Autodesk Inventor part; units mm, degrees
ref_plane "YZ Plane" through (0, 0, 0) normal (1, 0, 0) x (0, 1, 0)
ref_plane "XZ Plane" through (0, 0, 0) normal (0, 1, 0) x (-1, 0, 0)
ref_plane "XY Plane" through (0, 0, 0) normal (0, 0, 1) x (1, 0, 0)
sketch "Skizze1" plane through (0, 0, 0) normal (0, 1, 0) x (-1, 0, 0)
  arc A0 (112.1495, -122.8972) -> (112.1495, -22.8972) centre (112.1495, -72.8972) ccw
  circle A1 centre (8.4112, -73.6215) radius 17.5
  line L0 (112.1495, -122.8972) -> (8.4112, -91.1215)
  line L1 (112.1495, -22.8972) -> (8.4112, -56.1215)
  point P0 (0, 0)
  dimension "d0" = 50
  dimension "d1" = 35
extrude "Extrusion1" add sketch "Skizze1" along normal blind 10
sketch "Skizze2" plane through (0, 10, 0) normal (0, 1, 0) x (1, 0, 0)
  arc A0 (-112.1495, 122.8972) -> (-112.1495, 22.8972) centre (-112.1495, 72.8972) ccw
  circle A1 centre (-112.1495, 72.8972) radius 40
  point P0 (0, 0)
  dimension "d4" = 80
extrude "Extrusion2" add sketch "Skizze2" along normal blind 30
sketch "Skizze3" plane through (0, 0, 0) normal (0, -1, 0) x (1, 0, 0)
  circle A0 centre (-112.1495, -112.8972) radius 2.5
  circle A1 centre (-112.1495, -32.8972) radius 2.5
  circle A2 centre (1.5888, -73.3753) radius 2.5
  arc A3 (-8.4112, -91.1215) -> (-8.4112, -56.1215) centre (-8.4112, -73.6215) ccw
  circle A4 centre (-112.1495, -72.8972) radius 40
  point P0 (0, 0)
  dimension "d7" = 5
  dimension "d8" = 5
  dimension "d9" = 5
  dimension "d10" = 10
  dimension "d11" = 40
  dimension "d12" = 0
  dimension "d13" = 40
extrude "Extrusion3" add sketch "Skizze3" along normal blind 20 contours A0 A4 | A4 A0 | A4 A1 | A1 A4 | A2
properties part number "Sensor"
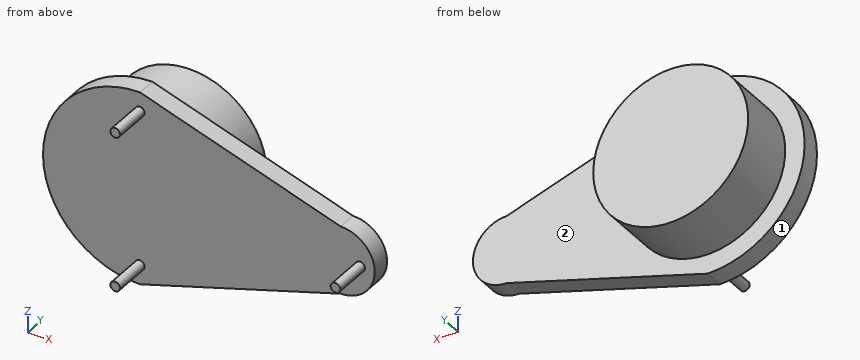
Input: part model. Units: mm. Frame: model coordinates. Face numbers are marked on the shaded views. A direction names the side the tool comes from. Coordinates: 2 decimals unless noted, no trailing zeros. Loops run counter-clockwise (first coordinate to the right, second up) from the corner with the lowest first, then second, coordinate; pieces in that order, holes last. Notation, with made-up numbers: (0.5, 36) -> (48.5, 36) arc R9 ccw to (48.5, 43) -> close; hole circle Ø11 at (-30.5, 52.5). An arc over 180 degrees is marked (long way). One line per item, written item: value.
(1) Pin query (flat end, axial travel): pin 1 Ø5 at (x, z) = (-76.5, -102) entering from -Y; pin 2 Ø8 at (x, y) = (-60, 15) entering from -Z; pin 3 Ø10 at (y, z) = (-11.5, -67) entering from -X; pin 4 Ø8 at (x, y) = (-142, -2) entering from +Z. Return the tip coordinate at first contact, or that it passes through.
Answer below:
pin 1: stops at y = 0
pin 2: passes through
pin 3: stops at x = -0.5
pin 4: stops at z = -30.43
(2) Ray query, line 1 along Y through (x, z) = (-32.5, -90); line 2 along Z through (x, y) = (-114, -12); line 3 along Y through (x, z) = (-134, -75.5). Return the intervals inside material, ascending.
Answer below:
line 1: y = 0 to 10
line 2: z = -114.58 to -111.22, -34.58 to -31.22
line 3: y = 0 to 40
(3) Cut plane A-A (x = -87). Output: boundary loops of the cut face in (y, z).
Answer below:
outline: (0, -115.19) -> (10, -115.19) -> (10, -104) -> (40, -104) -> (40, -41.79) -> (10, -41.79) -> (10, -30.95) -> (0, -30.95) -> close
(4) Cut plane B-B (z = -60.5). Output: boundary loops of the cut face in (x, y), then the cut area to 3 significant figures.
Answer below:
outline: (-160.59, 0) -> (3.17, 0) -> (3.17, 10) -> (-74.12, 10) -> (-74.12, 40) -> (-150.18, 40) -> (-150.18, 10) -> (-160.59, 10) -> close
area: 3,920 mm2
(5) Set-up query: the marked faces 1 and 2. Return all of +Z, -Z, +X, -X, +Y, -Y with unobstructed straight access to the full face (end or side cutting, diameter ignored); none if empty.
Answer below:
face 1: -X, +Y, -Y
face 2: +Y
(6) Cut plane C-C (y = 4.5). Output: boundary loops of the cut face in (x, z).
Answer below:
outline: (-112.15, -122.9) -> (-8.41, -91.12) arc R17.5 ccw to (-8.41, -56.12) -> (-112.15, -22.9) arc R50 ccw to start
(7) Cut plane D-D (x = -4.5). Output: boundary loops of the cut face in (y, z).
Answer below:
outline: (0, -90.68) -> (10, -90.68) -> (10, -56.56) -> (0, -56.56) -> close
